CAD build for the part. Positions are in the model's coordinates, mm. A direction names the side the tool comes from. Give positions to 0.01 mm unless a question says otherwise; leave off trailing zeros. Write each loop counter-clockwise with the first axis right and the second up, starting at its lowest first coordinate (ties: lowest second). Pieces come first, ordered by that corner, then holes. Notation, with made-up numbers: (57, -20.75) - (78, -20.75) arc R30 ccw to (78, 13.25) - close; hole circle Ø4 at (-39, 14). An arc over 180 degrees is marked (long way). Answer as a JSON object with one key per item and string values.
from build123d import *

# Parameters (mm, degrees)
SKETCH1_W           = 462
SKETCH1_H           = 292
BOSS_EXTRUDE1_DEPTH = 118
CHAMFER1_SIZE       = 30
CHAMFER1_SIZE2      = 10
SKETCH2_W           = 80
SKETCH2_H           = 40
BOSS_EXTRUDE2_DEPTH = 50
CUT_EXTRUDE1_DEPTH  = 293
SKETCH5_W           = 212
SKETCH5_H           = 83
CUT_EXTRUDE3_DEPTH  = 50
BOSS_EXTRUDE3_DEPTH = 30
BOSS_EXTRUDE5_REACH = 254
SHELL1_T            = -2.5
SKETCH9_R           = 7.5
CUT_EXTRUDE4_DEPTH  = 293


with BuildPart() as part:
    # Sketch1 → Boss-Extrude1 (new body)
    with BuildSketch(Plane(origin=(0, 0, 0), x_dir=(1, 0, 0), z_dir=(0, 1, 0))):
        Rectangle(SKETCH1_W, SKETCH1_H)
    extrude(amount=BOSS_EXTRUDE1_DEPTH)

    # Chamfer1
    chamfer1_edges = [part.edges().sort_by_distance(p)[0] for p in [
        (231, 0, 0),
    ]]
    chamfer1_side = [part.faces().sort_by_distance(p)[0] for p in [
        (0, 0, 0),
    ]]
    chamfer(chamfer1_edges, length=CHAMFER1_SIZE, length2=CHAMFER1_SIZE2, reference=chamfer1_side[0])

    # Sketch2 → Boss-Extrude2 (add)
    with BuildSketch(Plane(origin=(0, 118, 0), x_dir=(1, 0, 0), z_dir=(0, 1, 0))):
        with Locations((191, 126)):
            Rectangle(SKETCH2_W, SKETCH2_H)
        with Locations((191, -126)):
            Rectangle(SKETCH2_W, SKETCH2_H)
    extrude(amount=BOSS_EXTRUDE2_DEPTH)

    # Sketch3 → Cut-Extrude1 (cut, through all)
    with BuildSketch(Plane.XY.offset(146)):
        Polygon((151, 118), (196, 168), (151, 168), align=None)
    extrude(amount=-CUT_EXTRUDE1_DEPTH, mode=Mode.SUBTRACT)

    # Sketch5 → Cut-Extrude3 (cut)
    with BuildSketch(Plane(origin=(231, 0, 0), x_dir=(0, 0, -1), z_dir=(1, 0, 0))):
        with Locations((0, 76.5)):
            Rectangle(SKETCH5_W, SKETCH5_H)
    extrude(amount=-CUT_EXTRUDE3_DEPTH, mode=Mode.SUBTRACT)

    # Sketch6 → Boss-Extrude3 (add)
    with BuildSketch(Plane(origin=(199, 0, 0), x_dir=(0, 0, -1), z_dir=(1, 0, 0))):
        with BuildLine():
            Line((106, 165), (81.049437742, 165))
            ThreePointArc((81.049437742, 165), (79.312955966, 165.15192247), (77.629236309, 165.603073792))
            Line((77.629236309, 165.603073792), (38.656931626, 179.787832658))
            ThreePointArc((38.656931626, 179.787832658), (36.97321197, 180.23898398), (35.236730193, 180.39090645))
            Line((35.236730193, 180.39090645), (-35.236730193, 180.39090645))
            ThreePointArc((-35.236730193, 180.39090645), (-36.97321197, 180.23898398), (-38.656931626, 179.787832658))
            Line((-38.656931626, 179.787832658), (-77.629236309, 165.603073792))
            ThreePointArc((-77.629236309, 165.603073792), (-79.312955966, 165.15192247), (-81.049437742, 165))
            Line((-81.049437742, 165), (-106, 165))
            Line((-106, 165), (-106, 148))
            Line((-106, 148), (-81.049437742, 148))
            ThreePointArc((-81.049437742, 148), (-79.312955966, 148.15192247), (-77.629236309, 148.603073792))
            Line((-77.629236309, 148.603073792), (-38.656931626, 162.787832658))
            ThreePointArc((-38.656931626, 162.787832658), (-36.97321197, 163.23898398), (-35.236730193, 163.39090645))
            Line((-35.236730193, 163.39090645), (35.236730193, 163.39090645))
            ThreePointArc((35.236730193, 163.39090645), (36.97321197, 163.23898398), (38.656931626, 162.787832658))
            Line((38.656931626, 162.787832658), (77.629236309, 148.603073792))
            ThreePointArc((77.629236309, 148.603073792), (79.312955966, 148.15192247), (81.049437742, 148))
            Line((81.049437742, 148), (106, 148))
            Line((106, 148), (106, 165))
        make_face()
    extrude(amount=BOSS_EXTRUDE3_DEPTH)

    # Sketch8 → Boss-Extrude5 (add, up to next)
    with BuildSketch(Plane.XY.offset(-106), mode=Mode.PRIVATE) as boss_extrude5_sk1:
        Polygon((181, 112), (225.455970728, 35), (181, 35), align=None)
    boss_extrude5_tool1 = extrude(boss_extrude5_sk1.sketch, amount=BOSS_EXTRUDE5_REACH, mode=Mode.PRIVATE) - part.part
    add(boss_extrude5_tool1.solids().sort_by_distance((195.818657, 60.666667, -106))[0])

    # Shell1
    shell1_openings = [part.faces().sort_by_distance(p)[0] for p in [
        (-15, 0, 0),
    ]]
    offset(amount=SHELL1_T, openings=shell1_openings, kind=Kind.INTERSECTION)

    # Sketch9 → Cut-Extrude4 (cut, through all)
    with BuildSketch(Plane.XY.offset(146)):
        with Locations((-57, 59)):
            Circle(SKETCH9_R)
    extrude(amount=-CUT_EXTRUDE4_DEPTH, mode=Mode.SUBTRACT)


solid = part.part
Item 1: Mould opens along X. For faces 1 (the flat face through (213.79, 172.795, 57.87)), 2 (the flat face through (216, 5, 2)), 3 (the flat face through (213.825, 158.144, -58.725)) say: +X half, -X half, draft (parallel to the pull), parting line (faces both ways), or undercut.
Entries:
{"face 1": "draft", "face 2": "+X half", "face 3": "undercut"}
Item 2: Probe line 1 (Z direction, x = 196, y = 131); line 2 (Y direction, x = -57, z = 144.45); line 3 (Z direction, x = 142, y = 78.5). List the from-to ranges inside material, lowest first. Write a range as from..to.
Entries:
{"line 1": "-146..-143.5, -108.5..-106, 106..108.5, 143.5..146", "line 2": "0..51.5, 66.5..118", "line 3": "-146..-143.5, 143.5..146"}
Item 3: Cut at D-D (y = 59). Give the cut face in (x, z), and give its area (3 significant figures).
Entries:
{"outline": "(-231, -146) - (-64.5, -146) - (-64.5, -143.5) - (-228.5, -143.5) - (-228.5, 143.5) - (-64.5, 143.5) - (-64.5, 146) - (-231, 146) - close; (-49.5, -146) - (231, -146) - (231, -106) - (211.6, -106) - (211.6, 106) - (231, 106) - (231, 146) - (-49.5, 146) - (-49.5, 143.5) - (228.5, 143.5) - (228.5, 108.5) - (208.71, 108.5) - (208.71, -108.5) - (228.5, -108.5) - (228.5, -143.5) - (-49.5, -143.5) - close", "area": "3,850 mm2"}
Item 4: Flat gauge pins, fed straight in: P1, Ø7.5, axis at x = 207, z = -95, coming from the -Y side; P2, Ø6, axis at x = -38, z = -78.5, coming from the -Y side; P3, Ø15, axis at x = 218, z = -1.5, coming from the -Y side. Where does each tip first touch, or does it go through?
Entries:
{"P1": "y = 0.75", "P2": "y = 115.5", "P3": "y = 3.17"}
Item 5: Which spindle directions (+Z, -Z, +X, -X, +Y, -Y) get a long thin tool onto all of the face, cutting with end or side? Do faces 4 (the flat face through (211.04, 5.98, 2.01)), 5 (the flat face through (213, 168, -126)), 6 (the flat face through (229, 164, 1)). Say none if no direction does.
Entries:
{"face 4": "none", "face 5": "-Z, +X, -X, +Y", "face 6": "+X, +Y"}
Item 6: Cut at B-B (y = 134.5). Give the cut face in (x, z).
Entries:
{"outline": "(165.85, -146) - (231, -146) - (231, -106) - (165.85, -106) - close; (165.85, 106) - (231, 106) - (231, 146) - (165.85, 146) - close; hole (169.21, -143.5) - (228.5, -143.5) - (228.5, -108.5) - (169.21, -108.5) - close; hole (169.21, 108.5) - (228.5, 108.5) - (228.5, 143.5) - (169.21, 143.5) - close"}
Item 7: Cut at C-C (x = -57). Give the cut face in (y, z).
Entries:
{"outline": "(0, -146) - (51.5, -146) - (51.5, -143.5) - (0, -143.5) - close; (0, 143.5) - (51.5, 143.5) - (51.5, 146) - (0, 146) - close; (66.5, -146) - (118, -146) - (118, 146) - (66.5, 146) - (66.5, 143.5) - (115.5, 143.5) - (115.5, -143.5) - (66.5, -143.5) - close"}
Item 8: Cut at A-A (z = -29.5). Give the cut face in (x, y), and give its area (3 significant figures).
Entries:
{"outline": "(-231, 0) - (-228.5, 0) - (-228.5, 115.5) - (178.5, 115.5) - (178.5, 111.33) - (224.01, 32.5) - (228.5, 32.5) - (228.5, 11.8) - (193.09, 0) - (201, 0) - (231, 10) - (231, 35) - (225.46, 35) - (181, 112) - (181, 118) - (-231, 118) - close; (199, 163.39) - (229, 163.39) - (229, 180.39) - (199, 180.39) - close; hole (201.5, 165.89) - (226.5, 165.89) - (226.5, 177.89) - (201.5, 177.89) - close", "area": "1,920 mm2"}
